Autodesk Inventor part; units mm, degrees
ref_plane "YZ Plane" through (0, 0, 0) normal (1, 0, 0) x (0, 1, 0)
ref_plane "XZ Plane" through (0, 0, 0) normal (0, 1, 0) x (-1, 0, 0)
ref_plane "XY Plane" through (0, 0, 0) normal (0, 0, 1) x (1, 0, 0)
sketch "Sketch1" plane through (0, 0, 0) normal (0, 0, 1) x (1, 0, 0)
  circle A0 centre (0, 0) radius 26.4795
  dimension "d0" = 52.959
extrude "Extrusion1" add sketch "Sketch1" along normal blind 152.4
sketch "Sketch2" plane through (0, 0, 152.4) normal (0, 0, 1) x (1, 0, 0)
  circle A0 centre (0, 0) radius 13.97
  circle A1 centre (0, 0) radius 26.4795
  dimension "d3" = 27.94
extrude "Extrusion2" cut sketch "Sketch2" against normal blind 7.9248
sketch "Sketch3" plane through (0, 0, 0) normal (0, 0, -1) x (-1, 0, 0)
  circle A0 centre (0, 0) radius 13.97
  circle A1 centre (0, 0) radius 26.4795
  dimension "d6" = 27.94
extrude "Extrusion3" cut sketch "Sketch3" against normal blind 7.9248
sketch "Sketch4" plane through (0, 0, 7.9248) normal (0, 0, -1) x (-1, 0, 0)
  circle A0 centre (0, 0) radius 13.97
  circle A1 centre (0, 0) radius 25.2095
  circle A2 centre (0, 0) radius 26.4795
  dimension "d9" = 50.419
extrude "Extrusion4" cut sketch "Sketch4" against normal blind 116.84 contours A2
fillet "Fillet1" radius 1.27 1 edges at (-26.4795, 0, 124.7648)
chamfer "Chamfer1" distance 2.54 angle 78 1 edges at (-26.4795, 0, 144.4752) measured on face at (26.3936, -2.1307, 138.3282)
fillet "Fillet2" radius 1.27 1 edges at (-26.4795, 0, 141.9352)
chamfer "Chamfer2" distance 2.54 angle 77 1 edges at (25.2095, 0, 7.9248) measured on face at (-24.883, -4.0439, 85.8181)
fillet "Fillet3" radius 1.27 1 edges at (25.2095, 0, 10.4648)
sketch "Sketch6" plane through (0, 0, 152.4) normal (0, 0, 1) x (1, 0, 0)
  circle A0 centre (0, 0) radius 6.35
  dimension "d23" = 12.7
extrude "Extrusion6" cut sketch "Sketch6" against normal through all
sketch "Sketch7" plane through (0, 0, 7.9248) normal (0, 0, -1) x (-1, 0, 0)
  circle A0 centre (0, 0) radius 22.225
  dimension "d26" = 44.45
sketch "Sketch8" plane through (0, 0, 0) normal (0, 0, -1) x (-1, 0, 0)
  circle A0 centre (0, 0) radius 1.3033
extrude "Extrusion7" add sketch "Sketch8" against normal blind 76.2
sketch "Sketch9" plane through (0, 0, 76.2) normal (0, 0, 1) x (1, 0, 0)
  circle A0 centre (0, 0) radius 1.3033
  circle A1 centre (0, 0) radius 22.225
  dimension "d29" = 44.45
extrude "Extrusion8" cut sketch "Sketch9" along normal blind 63.5 and the other way blind 63.5
sketch "Sketch10" plane through (0, 0, 0) normal (0, 0, -1) x (-1, 0, 0)
  circle A0 centre (0, 0) radius 1.9784
extrude "Extrusion9" cut sketch "Sketch10" against normal through all
thread "Thread1"
thread "Thread2"
sketch "Sketch11" plane through (0, 0, 152.4) normal (0, 0, 1) x (1, 0, 0)
  circle A0 centre (0, 0) radius 12.7
  circle A1 centre (0, 0) radius 9.525
  circle A2 centre (0, 9.525) radius 1.5875
  circle A3 centre (9.525, 0) radius 1.5875
  circle A4 centre (0, -9.525) radius 1.5875
  circle A5 centre (-9.525, 0) radius 1.5875
  line L0 (-13.6194, 1.5875) -> (-8.6056, 1.5875)
  line L1 (-8.6056, 1.5875) -> (-8.6056, -1.5875)
  line L2 (-8.6056, -1.5875) -> (-13.6194, -1.5875)
  line L3 (-13.6194, -1.5875) -> (-13.6194, 1.5875)
  line L4 (-13.6194, 1.5875) -> (-8.6056, -1.5875) construction
  line L5 (-8.6056, 1.5875) -> (-13.6194, -1.5875) construction
  line L6 (6.086, 1.5875) -> (12.964, 1.5875)
  line L7 (12.964, 1.5875) -> (12.964, -1.5875)
  line L8 (12.964, -1.5875) -> (6.086, -1.5875)
  line L9 (6.086, -1.5875) -> (6.086, 1.5875)
  line L10 (6.086, 1.5875) -> (12.964, -1.5875) construction
  line L11 (12.964, 1.5875) -> (6.086, -1.5875) construction
  line L12 (-1.5875, -6.1744) -> (1.5875, -6.1744)
  line L13 (1.5875, -6.1744) -> (1.5875, -12.8756)
  line L14 (1.5875, -12.8756) -> (-1.5875, -12.8756)
  line L15 (-1.5875, -12.8756) -> (-1.5875, -6.1744)
  line L16 (-1.5875, -6.1744) -> (1.5875, -12.8756) construction
  line L17 (1.5875, -6.1744) -> (-1.5875, -12.8756) construction
  circle A6 centre (0, 0) radius 6.35
  line L18 (-1.5875, 12.9016) -> (1.5875, 12.9016)
  line L19 (1.5875, 12.9016) -> (1.5875, 6.1484)
  line L20 (1.5875, 6.1484) -> (-1.5875, 6.1484)
  line L21 (-1.5875, 6.1484) -> (-1.5875, 12.9016)
  line L22 (-1.5875, 12.9016) -> (1.5875, 6.1484) construction
  line L23 (1.5875, 12.9016) -> (-1.5875, 6.1484) construction
  point P0 (-11.1125, 0)
  point P1 (-1.5875, -9.3918)
  point P2 (-9.3918, -1.5875)
  point P3 (-12.6004, -1.5875)
  point P4 (-1.5875, -12.6004)
  point P5 (1.5875, -12.6004)
  point P6 (12.6004, -1.5875)
  point P7 (9.3918, -1.5875)
  point P8 (1.5875, -9.3918)
  point P9 (1.5875, 9.3918)
  point P10 (9.3918, 1.5875)
  point P11 (12.6004, 1.5875)
  point P12 (1.5875, 12.6004)
  point P13 (-1.5875, 12.6004)
  point P14 (-12.6004, 1.5875)
  point P15 (-9.3918, 1.5875)
  point P16 (-1.5875, 9.3918)
  dimension "d45" = 3.175
  dimension "d40" = 25.4
  dimension "d41" = 19.05
  dimension "d42" = 3.175
  dimension "d43" = 3.175
  dimension "d44" = 3.175
extrude "Extrusion10" cut sketch "Sketch11" against normal blind 6.35 contours L6 A1 L19 A0 | A0 L13 A1 L8 | L21 A1 L0 A0 | A0 L2 A1 L15
sketch "Sketch12" plane through (0, 0, 0) normal (0, 0, -1) x (-1, 0, 0)
  circle A0 centre (0, 0) radius 12.7
  line L0 (12.6004, -1.5875) -> (9.3918, -1.5875)
  circle A1 centre (0, 0) radius 9.525
  line L1 (-1.5875, 5.8819) -> (1.5875, 5.8819)
  line L2 (1.5875, 5.8819) -> (1.5875, 13.1681)
  line L3 (1.5875, 13.1681) -> (-1.5875, 13.1681)
  line L4 (-1.5875, 13.1681) -> (-1.5875, 5.8819)
  line L5 (-1.5875, 5.8819) -> (1.5875, 13.1681) construction
  line L6 (1.5875, 5.8819) -> (-1.5875, 13.1681) construction
  line L7 (5.4881, 1.5875) -> (13.5619, 1.5875)
  line L8 (13.5619, 1.5875) -> (13.5619, -1.5875)
  line L9 (13.5619, -1.5875) -> (5.4881, -1.5875)
  line L10 (5.4881, -1.5875) -> (5.4881, 1.5875)
  line L11 (5.4881, 1.5875) -> (13.5619, -1.5875) construction
  line L12 (13.5619, 1.5875) -> (5.4881, -1.5875) construction
  line L13 (-1.5875, -5.9212) -> (1.5875, -5.9212)
  line L14 (1.5875, -5.9212) -> (1.5875, -13.1288)
  line L15 (1.5875, -13.1288) -> (-1.5875, -13.1288)
  line L16 (-1.5875, -13.1288) -> (-1.5875, -5.9212)
  line L17 (-1.5875, -5.9212) -> (1.5875, -13.1288) construction
  line L18 (1.5875, -5.9212) -> (-1.5875, -13.1288) construction
  line L19 (-12.9783, 1.5875) -> (-6.0717, 1.5875)
  line L20 (-6.0717, 1.5875) -> (-6.0717, -1.5875)
  line L21 (-6.0717, -1.5875) -> (-12.9783, -1.5875)
  line L22 (-12.9783, -1.5875) -> (-12.9783, 1.5875)
  line L23 (-12.9783, 1.5875) -> (-6.0717, -1.5875) construction
  line L24 (-6.0717, 1.5875) -> (-12.9783, -1.5875) construction
  point P0 (0, 9.525)
  point P1 (9.525, 0)
  point P2 (0, -9.525)
  point P3 (-9.525, 0)
  point P4 (1.5875, -9.3918)
  point P5 (1.5875, -12.6004)
  point P6 (-9.3918, -1.5875)
  point P7 (-12.6004, -1.5875)
  point P8 (-1.5875, -12.6004)
  point P9 (-1.5875, -9.3918)
  point P10 (9.3918, 1.5875)
  point P11 (12.6004, 1.5875)
  point P12 (1.5875, 12.6004)
  point P13 (1.5875, 9.3918)
  point P14 (-12.6004, 1.5875)
  point P15 (-9.3918, 1.5875)
  point P16 (-1.5875, 9.3918)
  point P17 (-1.5875, 12.6004)
extrude "Extrusion11" cut sketch "Sketch12" against normal blind 6.35 contours A0 L14 A1 L0 | L7 A1 L2 A0 | A0 L21 A1 L16 | L4 A1 L19 A0
properties part number "2x6 Air Tank"
Here's how the part is built. I have some questions about the finished solid (model axes, mm). A direction names the side the tool comes from. Round coordinates to 2 decimals unless told otherwise and drop trailing zeros.
1. For faces 1 (the face through (5, -5, 12.7)), 2 (the face through (-1.588, 11, 149)), 3 (the face through (1.588, -11, 3)), 4 (the face through (-1.38, -6.2, 146.14)), which set-ups out of +Z, -Z, +X, -X, +Y, -Y let a thin tool reach every point of the face, with its end or its side?
Answers:
face 1: none
face 2: +Z
face 3: -Z
face 4: +Z, -Z
2. Thinking about a two-plate mould opening in Y: for faces 5 (the face through (-1.588, 11, 3)), 6 (the face through (8.9, 9.06, 3.13)), 7 (the face through (-11.91, 7.6, 144.475)), 8 (the face through (-1.82, 13.85, 148.49)), which applies, released by +Y, released by -Y, zero draft, split by the parting line, or undercut?
Answers:
face 5: undercut
face 6: undercut
face 7: zero draft
face 8: split by the parting line
3. If I drill on probe 1 along Z at (x, y) = (10.5, -4); probe 2 along X at (y, z) = (0.5, 123.5); probe 3 along Z at (x, y) = (0, 20), over which ranges is the centre line in solid material (lowest first)?
Answers:
probe 1: z = 6.35 to 12.7, 139.7 to 146.05
probe 2: x = -25.2 to -22.22, 22.22 to 25.2
probe 3: z = 9.26 to 12.7, 139.7 to 143.31
4. Will these pins go through, and if not, where does the flat tip stop? pin 1 (12 mm diameter, centred on x = 20, z = 28, fed in from -Y); pin 2 (8 mm diameter, centred on x = -5.5, z = 88, fed in from -Y); pin 3 (8 mm diameter, centred on y = 19, z = 43, fed in from -X).
Answers:
pin 1: stops at y = -20.96
pin 2: stops at y = -25.16
pin 3: stops at x = -20.26
